from build123d import *

# Parameters (mm, degrees)
SKETCH1_R                = 15.24
EXTRUDE1_DEPTH           = 106.68
EXTRUDE1_TAPER           = 3
EXTRUDE1_OTHER_WAY_DEPTH = 63.5
DOME1_FACE_RADIUS        = 15.24
DOME1_HEIGHT             = 15.24
EXTRUDE2_DEPTH           = 110.904540983
EXTRUDE2_DEPTH_BACK      = 110.904540983


with BuildPart() as part:
    # Sketch1 → Extrude1 (new body)
    with BuildSketch(Plane(origin=(0, 0, 0), x_dir=(0, 0, -1), z_dir=(1, 0, 0))):
        with Locations((0, 6.35)):
            Circle(SKETCH1_R)
    extrude(amount=EXTRUDE1_DEPTH, taper=EXTRUDE1_TAPER)

    # Sketch1 → Extrude1 other way (add)
    with BuildSketch(Plane(origin=(0, 0, 0), x_dir=(0, 0, -1), z_dir=(1, 0, 0))):
        with Locations((0, 6.35)):
            Circle(SKETCH1_R)
    extrude(amount=-EXTRUDE1_OTHER_WAY_DEPTH)

    # Dome1: a dome of height H over a round flat face of radius A is a cap of a sphere of radius (A * A + H * H) / (2 * H)
    dome1_r = (DOME1_FACE_RADIUS * DOME1_FACE_RADIUS + DOME1_HEIGHT * DOME1_HEIGHT) / (2 * DOME1_HEIGHT)
    dome1_base = Plane((-63.5, 6.35, 0), z_dir=(-1, 0, 0))
    with Locations(dome1_base.offset(DOME1_HEIGHT - dome1_r)):
        dome1_ball = Sphere(dome1_r, mode=Mode.PRIVATE)
    add(split(dome1_ball, bisect_by=dome1_base, keep=Keep.TOP, mode=Mode.PRIVATE))

    # Sketch3 → Extrude2 (cut, two sides: drawn at the far end of the back side and taken through both)
    with BuildSketch(Plane(origin=(0, 0, 0), x_dir=(0, 0, -1), z_dir=(1, 0, 0)).offset(-EXTRUDE2_DEPTH_BACK)):
        Polygon((0, 142.420252654), (0, 34.177667736), (0, -25.107363528), (0, -133.349948446), (216.485169836, -133.349948446), (216.485169836, 142.420252654), align=None)
    extrude(amount=EXTRUDE2_DEPTH + EXTRUDE2_DEPTH_BACK, mode=Mode.SUBTRACT)


solid = part.part
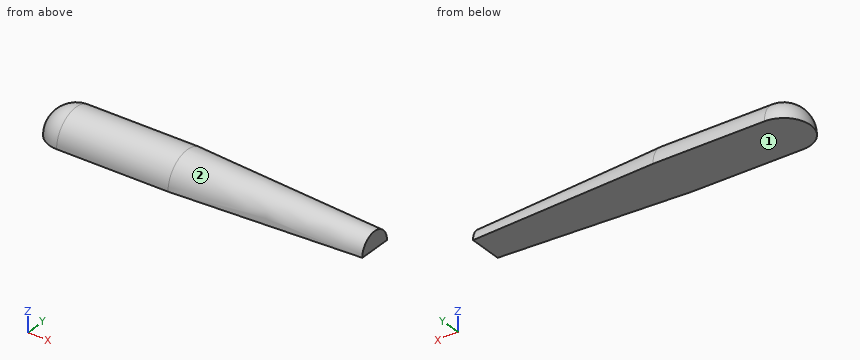
Design review of the part built by this model. Coordinates are the model's own, in mm. Face numbers are marked on the shaded views. Give positions to 0.01 mm unless a question says otherwise; leave off trailing zeros. Write each loop counter-clockwise with the first axis right and the second up, starting at its lowest first coordinate (ties: lowest second). Pieces come first, ordered by that corner, then holes. Notation, with made-up numbers: M 66,27 L 123,27 A8 cw 123,36 Z; hole C 0,0 d10. An arc over 180 degrees is marked long. Return JSON: item names as keys, results as strings. Group by question number.
Item 1: The part is to be moulded in two halves that separate along Z. For the marked faces 1 and 2, say which applies: pulls with the +Z half, pulls with the -Z half, needs draft (parallel to the pull), parting line crosses it, or undercut.
Item 2: Clearance check with flat-ended pins moving along their axes: pin 1 Ø6 at (y, z) = (11.5, 11.5) entering from +X; pin 2 Ø5 at (x, z) = (64, 13) entering from +Y; pin 3 Ø4 at (x, z) = (85, 10.5) entering from +Y; pin 4 Ø1 at (x, z) = (80.5, 4) entering from +Y. State where each tip first meets the part, or that it passes through.
Item 3: Take a section at C-C (x = 89.5). Give the boundary of the cut face in (y, z), plus the area to 3 significant figures.
Item 4: Wall thickness on line 1 along X through (y, z) = (2.5, 1.5); line 2 along Y through (x, z) = (-1, 3); line 3 along Z through (x, y) = (-10.5, -0.5): over which ranges is each line inside the solid? List them lowest first.
Item 5: Take a section at B-B (x = -21). Give the boundary of the cut face in (y, z).
Item 6: Take a section at A-A (y = 6.35). Give the boundary of the cut face in (x, z), plus the area to 3 significant figures.
Return value:
{
 "1": {"face 1": "pulls with the -Z half", "face 2": "pulls with the +Z half"},
 "2": {"pin 1": "stops at x = 106.68", "pin 2": "stops at y = 11.93", "pin 3": "stops at y = 12.99", "pin 4": "stops at y = 16.8"},
 "3": {"outline": "M -4.2,0 L 16.9,0 A10.55 ccw Z", "area": "175 mm2"},
 "4": {"line 1": "x = -78.17 to 106.68", "line 2": "y = -8.59 to 21.29", "line 3": "z = 0 to 13.61"},
 "5": {"outline": "M -8.89,0 L 21.59,0 A15.24 ccw Z"},
 "6": {"outline": "M -78.74,0 L 106.68,0 L 106.68,9.65 L 0,15.24 L -63.5,15.24 A15.24 ccw Z", "area": "2,480 mm2"}
}
